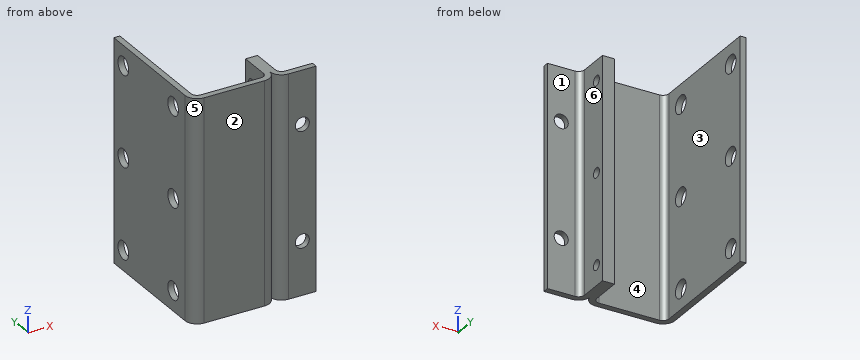
from build123d import *

# Parameters (mm, degrees)
F1_DEPTH      = 55
F1_DEPTH_BACK = 55
F2_R          = 2.5
F3_DEPTH      = 45.001
F4_R          = 4.5
F5_DEPTH      = 3
F6_R          = 4.5
F7_DEPTH      = 3
F8_R          = 3.5
F9_DEPTH      = 3


with BuildPart() as f1:
    # F0 (on Top) → F1 (new body, two sides)
    with BuildSketch(Plane.XY) as f1_sk:
        with BuildLine():
            Line((-39, 45), (-42, 45))
            Line((-42, 45), (-42, -15))
            ThreePointArc((-42, -15), (-40.242641, -19.242641), (-36, -21))
            Line((-36, -21), (-6, -21))
            ThreePointArc((-6, -21), (-1.757359, -19.242641), (0, -15))
            ThreePointArc((0, -15), (1.757359, -19.242641), (6, -21))
            Line((6, -21), (19.739676, -21))
            Line((19.739676, -21), (19.739676, -18))
            Line((19.739676, -18), (6, -18))
            ThreePointArc((6, -18), (3.87868, -17.12132), (3, -15))
            Line((3, -15), (3, 0))
            Line((3, 0), (-3, 0))
            Line((-3, 0), (-3, -15))
            ThreePointArc((-3, -15), (-3.87868, -17.12132), (-6, -18))
            Line((-6, -18), (-36, -18))
            ThreePointArc((-36, -18), (-38.12132, -17.12132), (-39, -15))
            Line((-39, -15), (-39, 45))
        make_face()
    extrude(amount=F1_DEPTH)
    extrude(f1_sk.sketch, amount=-F1_DEPTH_BACK)

    # F2 (on face) → F3 (cut, through all)
    with BuildSketch(Plane.YZ.offset(3)):
        with Locations((-5, 45)):
            Circle(F2_R)
        with Locations((-5, 0)):
            Circle(F2_R)
        with Locations((-5, -45)):
            Circle(F2_R)
    extrude(amount=-F3_DEPTH, mode=Mode.SUBTRACT)

    # F4 (on face) → F5 (cut)
    with BuildSketch(Plane.YZ.offset(-39)):
        with Locations((-5, 45)):
            Circle(F4_R)
        with Locations((-5, 0)):
            Circle(F4_R)
        with Locations((-5, -45)):
            Circle(F4_R)
    extrude(amount=-F5_DEPTH, mode=Mode.SUBTRACT)

    # F6 (on face) → F7 (cut)
    with BuildSketch(Plane.YZ.offset(-39)):
        with Locations((37, 0)):
            Circle(F6_R)
        with Locations((37, -45)):
            Circle(F6_R)
        with Locations((37, 45)):
            Circle(F6_R)
    extrude(amount=-F7_DEPTH, mode=Mode.SUBTRACT)

    # F8 (on face) → F9 (cut)
    with BuildSketch(Plane.XZ.offset(21)):
        with Locations((12.85351, 28.5)):
            Circle(F8_R)
        with Locations((12.85351, -28.5)):
            Circle(F8_R)
    extrude(amount=-F9_DEPTH, mode=Mode.SUBTRACT)


solid = f1.part
The listing builds one solid part. Answer for the finished solid, in the listing's coordinates (mm). Face numbers are marked on the shaded views. A direction names the side the tool comes from. Round coordinates to 2 decimals unless told otherwise and drop trailing zeros. Write each loop counter-clockwise with the first axis right and the second up, starting at its lowest first coordinate (ties: lowest second). Pieces come first, ordered by that corner, then holes. Notation, with made-up numbers: M -15.75,-25.5 L 26.25,-25.5 A12 ccw 26.25,-2.5 Z; hole C -1.5,-24 d4. An arc over 180 degrees is marked long. Write each question's results on one line, items separated by ' | '. Start each with the question number.
(1) For the marked faces 4, 5 and 6, determine the directions among +Z, -Z, +X, -X, +Y, -Y from which every point of the face is accessible in a straight line to the end or side of a thin tool.
(2) The part is cut by section B-B, the plane z = -45. Give the number of separate pieces and of enclosed holes in the cut face, and give its area (3 significant figures).
(3) Determine the mould class of the marked faces 1, 2 and 3 for opening direction Y: +Y half, -Y half, draft (parallel to the pull), parting line (faces both ways), or undercut.
(4) The part is cut by section C-C, the plane z = 28.5. Write down the section's boundary in (x, y), and give its area (3 significant figures).
(5) The part is cut by section A-A, the plane y = 37. Write down the section's boundary in (x, z).
(6) Find the intervals of material crossed by line 1 (Z direction, x = -40.8, y = -5); line 2 (X direction, y = -19, z = 28); line 3 (X direction, y = 33, z = 29.5), in increasing order.
(7) Each of these flat-tipped pins is pushed along its axis until it touches: P1, Ø11, axis at x = 12.85, z = -28.5, coming from the +Y side; P2, Ø3, axis at y = 21.5, z = -42.5, coming from the +X side; P3, Ø8, axis at y = -5, z = 0, coming from the -X side; P4, Ø4, axis at x = 12.85, z = 28.5, coming from the -Y side. Where does it stop, or does it pass through?
(8) The part is cut by section D-D, the plane z = -8.5. Write down the section's boundary in (x, y).
Worked answers:
1) face 4: +Z, -Z, +Y | face 5: +Z, -Z, -X, -Y | face 6: +Z, -Z, +X, +Y
2) separate pieces: 4 | enclosed holes: 0 | area: 381 mm²
3) face 1: +Y half | face 2: -Y half | face 3: draft
4) outline: M -42,-15 A6 ccw -36,-21 L -6,-21 A6 ccw 0,-15 A6 ccw 6,-21 L 9.35,-21 L 9.35,-18 L 6,-18 A3 cw 3,-15 L 3,0 L -3,0 L -3,-15 A3 cw -6,-18 L -36,-18 A3 cw -39,-15 L -39,45 L -42,45 Z; M 16.35,-21 L 19.74,-21 L 19.74,-18 L 16.35,-18 Z | area: 444 mm²
5) outline: M -42,-55 L -39,-55 L -39,-49.5 L -42,-49.5 Z; M -42,-40.5 L -39,-40.5 L -39,-4.5 L -42,-4.5 Z; M -42,4.5 L -39,4.5 L -39,40.5 L -42,40.5 Z; M -42,49.5 L -39,49.5 L -39,55 L -42,55 Z
6) line 1: z = -55 to -49.5, -40.5 to -4.5, 4.5 to 40.5, 49.5 to 55 | line 2: x = -40.47 to -1.53, 1.53 to 9.39, 16.32 to 19.74 | line 3: x = -42 to -39
7) P1: stops at y = -18 | P2: stops at x = -39 | P3: stops at x = -3 | P4: passes through
8) outline: M -42,-15 A6 ccw -36,-21 L -6,-21 A6 ccw 0,-15 A6 ccw 6,-21 L 19.74,-21 L 19.74,-18 L 6,-18 A3 cw 3,-15 L 3,0 L -3,0 L -3,-15 A3 cw -6,-18 L -36,-18 A3 cw -39,-15 L -39,45 L -42,45 Z
